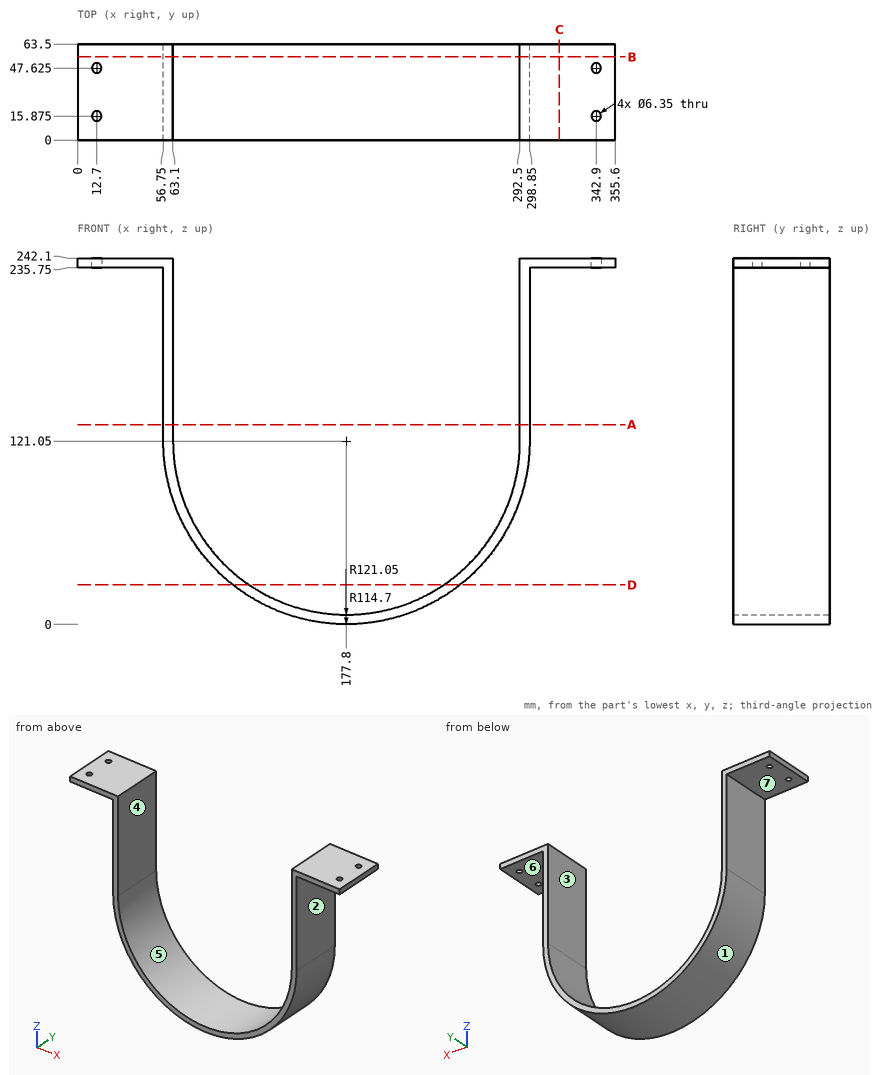
Input: dimensioned drawing with shaded views. Units: mm. Origin: part minimum x, y, z. A direction names the side the tool comes from. Coordinates: 2 decimals unless noted, no trailing zeros. Loops run counter-clockwise (first coordinate to the right, second up) from the corner with the lowest first, then second, coordinate; pieces in that order, holes last. Notation, with made-up numbers: M 44,53.5 L 70,53.5 A16 ccw 70,73.5 Z; hole C -12,68.25 d4. An arc over 180 degrees is marked long. Use a Markdown table: item, result. Add a question column.
1) Draft query along X for the marked faces 1, 2, 3 and 4. Return one class per face: +X half, -X half, draft (parallel to the pull), parting line (faces both ways), or undercut.
2) Section D-D, the plane z = 26. Return the cut outline in (x, y), plus the area to 3 significant figures.
3) Pin query (flat end, axial travel): P1, Ø6, axis at x = 253, y = 37.5, coming from the -Z side; P2, Ø3, axis at x = 120.5, y = 20, coming from the -Z side; P3, Ø4, axis at x = 342.9, y = 47.625, coming from the -Z side; P4, Ø3, axis at y = 20.5, z = 136.5, coming from the +X side. Return the tip coordinate at first contact, or that it passes through.
4) Section A-A, the plane z = 132. Return the cut outline in (x, y).
5) Set-up query: the marked faces 5, 6 and 7. Return all of +Z, -Z, +X, -X, +Y, -Y with unobstructed straight access to the full face (end or side cutting, diameter ignored); none if empty.
6) Section B-B, the plane y = 55. Return the cut outline in (x, z).
7) Section C-C, the plane x = 318.5. Return the cut outline in (y, z).
8) Line query: L1, parallel to Y at x = 12.7, z = 239.75; L2, parallel to Y at x = 12, z = 239; L3, parallel to X at y = 26, z = 231.5. Output: solid intervals per line, ascending. Write a range as from..to.
Answer below:
| question | item | result |
|---|---|---|
| 1 | face 1 | parting line |
| 1 | face 2 | +X half |
| 1 | face 3 | undercut |
| 1 | face 4 | undercut |
| 2 | outline | M 102.84,0 L 113.6,0 L 113.6,63.5 L 102.84,63.5 Z; M 242,0 L 252.76,0 L 252.76,63.5 L 242,63.5 Z |
| 2 | area | 1,370 mm2 |
| 3 | P1 | z = 23.89 |
| 3 | P2 | z = 13.63 |
| 3 | P3 | through |
| 3 | P4 | x = 298.85 |
| 4 | outline | M 56.75,0 L 63.1,0 L 63.1,63.5 L 56.75,63.5 Z; M 292.5,0 L 298.85,0 L 298.85,63.5 L 292.5,63.5 Z |
| 5 | face 5 | +Z, +Y, -Y |
| 5 | face 6 | -Z, +X, +Y, -Y |
| 5 | face 7 | -Z, -X, +Y, -Y |
| 6 | outline | M 0,235.75 L 56.75,235.75 L 56.75,121.05 A121.05 ccw 298.85,121.05 L 298.85,235.75 L 355.6,235.75 L 355.6,242.1 L 292.5,242.1 L 292.5,121.05 A114.7 cw 63.1,121.05 L 63.1,242.1 L 0,242.1 Z |
| 7 | outline | M 0,235.75 L 63.5,235.75 L 63.5,242.1 L 0,242.1 Z |
| 8 | L1 | 0..12.7, 19.05..44.45, 50.8..63.5 |
| 8 | L2 | 0..12.78, 18.97..44.53, 50.72..63.5 |
| 8 | L3 | 56.75..63.1, 292.5..298.85 |
